from build123d import *

# Parameters (mm, degrees)
EXTRUDE_1_DEPTH     = 4
SKETCH_2_R          = 1.6
CUT_EXTRUDE_1_DEPTH = 92.38927727
SKETCH_3_R          = 2.6
SKETCH_3_R_2        = 1.6
CUT_EXTRUDE_2_DEPTH = 92.38927727
FILLET_1_R          = 7


with BuildPart() as part:
    # 草图1 → 凸台-拉伸1 (new body)
    with BuildSketch(Plane(origin=(0, 0, 0), x_dir=(1, 0, 0), z_dir=(0, 1, 0))):
        Polygon((25, 0), (-25, 0), (-80, 29), (-80, 44), (80, 44), (80, 29), align=None)
    extrude(amount=EXTRUDE_1_DEPTH)

    # 草图2 → 切除-拉伸1 (cut, through all)
    with BuildSketch(Plane(origin=(0, 4, 0), x_dir=(1, 0, 0), z_dir=(0, 1, 0))):
        with Locations(Location((-7.5, 28, 0), (0, 0, 270))):
            Circle(SKETCH_2_R)
        with Locations(Location((7.5, 28, 0), (0, 0, 90))):
            Circle(SKETCH_2_R)
        with Locations(Location((-7.5, 12, 0), (0, 0, 90))):
            Circle(SKETCH_2_R)
        with Locations(Location((7.5, 12, 0), (0, 0, 270))):
            Circle(SKETCH_2_R)
    extrude(amount=-CUT_EXTRUDE_1_DEPTH, mode=Mode.SUBTRACT)

    # 草图3 → 切除-拉伸2 (cut, through all)
    with BuildSketch(Plane(origin=(0, 4, 0), x_dir=(1, 0, 0), z_dir=(0, 1, 0))):
        with Locations(Location((-73, 36, 0), (0, 0, 270))):
            Circle(SKETCH_3_R)
        with Locations(Location((73, 36, 0), (0, 0, 90))):
            Circle(SKETCH_3_R)
        with Locations(Location((-13.5, 17, 0), (0, 0, 270))):
            Circle(SKETCH_3_R_2)
        with Locations(Location((-13.5, 37, 0), (0, 0, 270))):
            Circle(SKETCH_3_R_2)
        with Locations(Location((13.5, 17, 0), (0, 0, 90))):
            Circle(SKETCH_3_R_2)
        with Locations(Location((13.5, 37, 0), (0, 0, 90))):
            Circle(SKETCH_3_R_2)
        with BuildLine():
            Line((-66, 37.045901786), (-66, 27.918180848))
            ThreePointArc((-66, 27.918180848), (-65.839389964, 27.374651191), (-65.409151024, 27.005714169))
            Line((-65.409151024, 27.005714169), (-31.946763962, 12.00114442))
            ThreePointArc((-31.946763962, 12.00114442), (-30.671368472, 12.413990718), (-30.952679882, 13.724692673))
            Line((-30.952679882, 13.724692673), (-64.415066944, 37.85698336))
            ThreePointArc((-64.415066944, 37.85698336), (-65.455558418, 37.936107677), (-66, 37.045901786))
        make_face()
        with BuildLine():
            Line((-53.712306987, 37.53593293), (-33.713971886, 23.113601522))
            ThreePointArc((-33.713971886, 23.113601522), (-32.673480412, 23.034477205), (-32.12903883, 23.924683096))
            Line((-32.12903883, 23.924683096), (-32.12903883, 35.147280888))
            ThreePointArc((-32.12903883, 35.147280888), (-32.368121456, 35.796129676), (-32.971048329, 36.13472152))
            Line((-32.971048329, 36.13472152), (-52.96938343, 39.334455136))
            ThreePointArc((-52.96938343, 39.334455136), (-54.051625259, 38.728799106), (-53.712306987, 37.53593293))
        make_face()
        with BuildLine():
            Line((-21.676324022, 7.610054966), (-25.148014353, 25.176303846))
            ThreePointArc((-25.148014353, 25.176303846), (-26.22644397, 25.97766474), (-27.12903883, 24.982419926))
            Line((-27.12903883, 24.982419926), (-27.12903883, 10.309246321))
            ThreePointArc((-27.12903883, 10.309246321), (-27.034628251, 9.885090925), (-26.76922323, 9.541025042))
            Line((-26.76922323, 9.541025042), (-23.2975329, 6.647949766))
            ThreePointArc((-23.2975329, 6.647949766), (-22.147000978, 6.556202787), (-21.676324022, 7.610054966))
        make_face()
        with BuildLine():
            Line((26.76922323, 9.541025042), (23.2975329, 6.647949766))
            ThreePointArc((23.2975329, 6.647949766), (22.147000978, 6.556202787), (21.676324022, 7.610054966))
            Line((21.676324022, 7.610054966), (25.148014353, 25.176303846))
            ThreePointArc((25.148014353, 25.176303846), (26.22644397, 25.97766474), (27.12903883, 24.982419926))
            Line((27.12903883, 24.982419926), (27.12903883, 10.309246321))
            ThreePointArc((27.12903883, 10.309246321), (27.034628251, 9.885090925), (26.76922323, 9.541025042))
        make_face()
        with BuildLine():
            Line((32.971048329, 36.13472152), (52.96938343, 39.334455136))
            ThreePointArc((52.96938343, 39.334455136), (54.051625259, 38.728799106), (53.712306987, 37.53593293))
            Line((53.712306987, 37.53593293), (33.713971886, 23.113601522))
            ThreePointArc((33.713971886, 23.113601522), (32.673480412, 23.034477205), (32.12903883, 23.924683096))
            Line((32.12903883, 23.924683096), (32.12903883, 35.147280888))
            ThreePointArc((32.12903883, 35.147280888), (32.368121456, 35.796129676), (32.971048329, 36.13472152))
        make_face()
        with BuildLine():
            Line((30.952679882, 13.724692673), (64.415066944, 37.85698336))
            ThreePointArc((64.415066944, 37.85698336), (65.455558418, 37.936107677), (66, 37.045901786))
            Line((66, 37.045901786), (66, 27.918180848))
            ThreePointArc((66, 27.918180848), (65.839389964, 27.374651191), (65.409151024, 27.005714169))
            Line((65.409151024, 27.005714169), (31.946763962, 12.00114442))
            ThreePointArc((31.946763962, 12.00114442), (30.671368472, 12.413990718), (30.952679882, 13.724692673))
        make_face()
    extrude(amount=-CUT_EXTRUDE_2_DEPTH, mode=Mode.SUBTRACT)

    # 圆角1
    fillet_1_edges = [part.edges().sort_by_distance(p)[0] for p in [
        (-80, 2, -29),
        (-80, 2, -44),
        (80, 2, -44),
        (80, 2, -29),
        (25, 2, 0),
        (-25, 2, 0),
    ]]
    fillet(fillet_1_edges, radius=FILLET_1_R)


solid = part.part
Verification items for the finished model (mm, model axes). A direction names the side the tool comes from. Coordinates: 2 decimals unless noted, no trailing zeros. Write each loop counter-clockwise with the first axis right and the second up, starting at its lowest first coordinate (ties: lowest second). Pieces come first, ordered by that corner, then holes. Notation, with made-up numbers: M 71,18.5 L 87,18.5 A15 ccw 87,36.5 Z; hole C 59,4 d2. An arc over 180 degrees is marked long. One line per question, with ' | ' between items.
1) Sectioned sample at D-D on z = -3.5. Record the cut outline in (x, y).
Solutions:
outline: M -31.64,0 L 31.64,0 L 31.64,4 L -31.64,4 Z
2) Sectioned sample at A-A on x = 7.5. Record the cut outline in (y, z).
Solutions:
outline: M 0,-44 L 4,-44 L 4,-29.6 L 0,-29.6 Z; M 0,-26.4 L 4,-26.4 L 4,-13.6 L 0,-13.6 Z; M 0,-10.4 L 4,-10.4 L 4,0 L 0,0 Z
3) Material ranges on L1, parallel to Z at x = 13.5, y = 2.9; L2, parallel to X at y = 3.25, z = -21; L3, parallel to Z at x = 44.5, y = 1.55, recorded low to high.
Solutions:
L1: -44 to -38.6, -35.4 to -18.6, -15.4 to 0 | L2: -64.83 to -52.02, -41.04 to -27.13, -24.32 to 24.32, 27.13 to 41.04, 52.02 to 64.83 | L3: -44 to -37.98, -30.89 to -23.49, -17.63 to -10.28
4) Access from +Z, -Z, +X, -X, +Y, -Y to the whole of each face (thin tool, end or side, straight path). Record for faces 1 (the face through (-51.051, 1.972, -13.736)), 2 (the face through (47.45, 2.03, -25.62)).
Solutions:
face 1: +Z, -X, +Y, -Y | face 2: +Y, -Y
5) Release check for a two-part mould opening along X. For faces 3 (the face through (-32.129, 2, -29)), 4 (the face through (-78.966, 2.028, -29.561)), 5 (the face through (-1, 2, -44)) record: +X half, -X half, draft (parallel to the pull), parting line (faces both ways), or undercut.
Solutions:
face 3: undercut | face 4: -X half | face 5: draft
6) Sectioned sample at C-C on x = -48. Record the cut outline in (y, z), then the cut area to 3 significant figures.
Solutions:
outline: M 0,-44 L 4,-44 L 4,-38.54 L 0,-38.54 Z; M 0,-33.42 L 4,-33.42 L 4,-26.02 L 0,-26.02 Z; M 0,-19.2 L 4,-19.2 L 4,-12.13 L 0,-12.13 Z | area: 79.7 mm^2
7) Depth check by flat-ended pin: pin 1 Ø5 at (x, z) = (-7.5, -28) entering from +Y; pin 2 Ø2 at (y, z) = (1.5, -28.5) entering from -X; pin 3 Ø1.9 at (x, z) = (7.5, -12) entering from +Y; pin 4 Ø2 at (y, z) = (2, -30.5) entering from +X. Enter the tip coordinate at first touch or a pass-through.
Solutions:
pin 1: y = 4 | pin 2: x = -78.93 | pin 3: through | pin 4: x = 79.78
8) Sectioned sample at B-B on y = 1.75. State how many separate pieces and enclosed holes the cut face has, then the cut area to 3 significant figures.
Solutions:
separate pieces: 1 | enclosed holes: 16 | area: 4,350 mm^2
